Geometry: see drawing. Coordinates: mm, zero at the bounding-box minimum. A direction names the side the tool comes from. Round coordinates to 2 decimals unless told otherwise and drop trailing zeros. Loops run counter-clockwise (first coordinate to the right, second up) from the corner with the lowest first, then second, coordinate; pieces in that order, holes last. Notation, with made-up numbers: (18.25, 58.5) -> (72.25, 58.5) arc R32 ccw to (72.25, 94.5) -> close; hole circle Ø10 at (61, 10). An arc over 180 degrees is marked (long way). Write item = value, one per line.
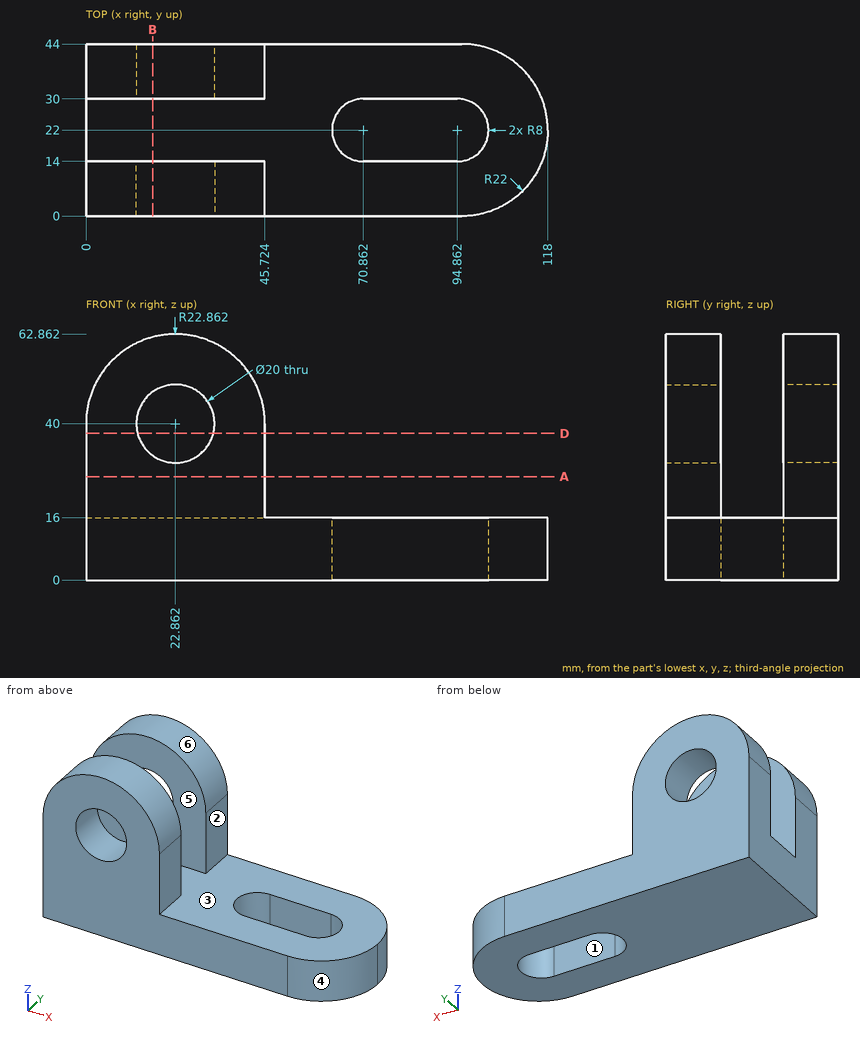
1. Mould query, pull axis Y, two halves, no side actions, for the marked faces 4, 5 and 6. Classes: released by +Y, released by -Y, zero draft, split by the parting line, or undercut.
Evaluation:
face_4 = released by -Y
face_5 = undercut
face_6 = zero draft
2. Section query A-A (z = 26.5). Return the cut outline in (x, y), then the cut area to 3 significant figures.
Evaluation:
outline = (0, 0) -> (45.72, 0) -> (45.72, 14) -> (0, 14) -> close; (0, 30) -> (45.72, 30) -> (45.72, 44) -> (0, 44) -> close
area = 1,280 mm²
3. Section query D-D (z = 37.5). Return the cut outline in (x, y) (1 decimal), then the cut area to 3 significant figures.
Evaluation:
outline = (0, 0) -> (13.2, 0) -> (13.2, 14) -> (0, 14) -> close; (0, 30) -> (13.2, 30) -> (13.2, 44) -> (0, 44) -> close; (32.5, 0) -> (45.7, 0) -> (45.7, 14) -> (32.5, 14) -> close; (32.5, 30) -> (45.7, 30) -> (45.7, 44) -> (32.5, 44) -> close
area = 738 mm²
4. Set-up query: the marked faces 1, 2 and 3. Return all of +Z, -Z, +X, -X, +Y, -Y with unobstructed straight access to the full face (end or side cutting, diameter ignored); none if empty.
Evaluation:
face_1 = +Z, -Z
face_2 = +Z, +X, +Y, -Y
face_3 = +Z, +X
5. Line query: probe 1 along Y at (x, z) = (38.5, 35); probe 2 along X at (y, z) = (23.5, 11.5); probe 3 along Z at (x, y) = (31, 37) (1 decimal). Output: solid intervals per line, ascending. Write a range as from..to.
Evaluation:
probe_1 = 0..14, 30..44
probe_2 = 0..63, 102.72..117.95
probe_3 = 0..34.2, 45.8..61.4
6. Section query B-B (x = 17). Return the cut outline in (y, z).
Evaluation:
outline = (0, 0) -> (44, 0) -> (44, 31.9) -> (30, 31.9) -> (30, 16) -> (14, 16) -> (14, 31.9) -> (0, 31.9) -> close; (0, 48.1) -> (14, 48.1) -> (14, 62.1) -> (0, 62.1) -> close; (30, 48.1) -> (44, 48.1) -> (44, 62.1) -> (30, 62.1) -> close
7. Contact query for flat-ended pins moving along their axis: pin 1 Ø4 at (y, z) = (5, 27.5) entering from +X; pin 2 Ø13 at (x, y) = (35, 18) entering from +Z; pin 3 Ø5 at (x, y) = (20.5, 19.5) entering from +Z. Output: stop coordinate, or through.
Evaluation:
pin_1 = 45.72
pin_2 = 61.76
pin_3 = 16
